```python
from build123d import *

# Parameters (mm, degrees)
F1_DEPTH = 9.525
F2_R     = 5.08
F3_R     = 5.08
F4_R     = 5.08
F5_R     = 7.06815
F6_DEPTH = 75.62089


with BuildPart() as f1:
    # F0 (on Top) → F1 (new body)
    with BuildSketch(Plane.XY):
        Polygon((36.595166, -42.144418), (55.044204, -31.628042), (-28.496206, 58.19229), (-68.840876, 46.343863), (-45.743927, 16.047873), align=None)
    extrude(amount=F1_DEPTH)

    # F2
    f2_edges = [f1.edges().sort_by_distance(p)[0] for p in [
        (-68.840876, 46.343863, 4.7625),
    ]]
    fillet(f2_edges, radius=F2_R)

    # F3
    f3_edges = [f1.edges().sort_by_distance(p)[0] for p in [
        (36.595166, -42.144418, 4.7625),
    ]]
    fillet(f3_edges, radius=F3_R)

    # F4
    f4_edges = [f1.edges().sort_by_distance(p)[0] for p in [
        (55.044204, -31.628042, 4.7625),
    ]]
    fillet(f4_edges, radius=F4_R)

    # F5 (on face) → F6 (cut)
    with BuildSketch(Plane(origin=(0, 0, 0), x_dir=(1, 0, 0), z_dir=(0, 0, -1))):
        with Locations((36.157202, 27.517132)):
            Circle(F5_R)
    extrude(amount=-F6_DEPTH, mode=Mode.SUBTRACT)


solid = f1.part
```
Verification items for the finished model (mm, model axes). Round coordinates to 2 decimals unless told otherwise and drop trailing zeros. Order: outer loops, then holes, each group sorted by start corner. A loop starts at its lowest first (then second) coordinate and runs counter-clockwise, first axis right, second up. Notation, with made-up numbers: (73.5, 35.5) - (98.5, 35.5) arc R19 ccw to (98.5, 66.5) - close; hole circle Ø10 at (-4, -19). An arc over 180 degrees is marked (long way). Use CSV: the item, a comma, the result in double quotes. Start each with the question number.
1) Go/stop test with flat-tipped pins: P1, Ø5, axis at x = 3, z = 1, coming from the -Y side; P2, Ø5, axis at y = 46, z = 6.5, coming from the +X side; P3, Ø22.5, axis at x = 36.16, y = -27.52, coming from the -Z side. Record where each tip stops, or that it passes through.
2) Section check B-B, the plane y = 28.5. Record the cut outline in (x, z) (3 decimals), plus the area to 3 significant figures.
3) Section check C-C, the plane x = -10. Record the cut outline in (y, z) (3 decimals), plus the area to 3 significant figures.
4) Thickness scan on L1, parallel to Y at x = 41, z = 2.75; L2, parallel to Y at x = 36, z = 5.25; L3, parallel to X at y = -30, z = 4.5. Record the ranges inside material, lowest first.
5) Section check A-A, the plane z = 2. Record the cut outline in (x, y).
6) Mould release check, pull along X, two halves, no side actions. Record for faces 1 (the flat face through (44.367, -37.714, 4.696)), 2 (the cylindrical face through (36.681, -41.206, 4.829)), 3 (the cylindrical face through (30.548, -23.216, 4.696)): +X half, -X half, draft (parallel to the pull), parting line (faces both ways), or undercut.
Answers:
1,P1,"stops at y = -20.17"
1,P2,"stops at x = -14.83"
1,P3,"stops at z = 0"
2,outline,"(-55.237, 0) - (-0.88, 0) - (-0.88, 9.525) - (-55.237, 9.525) - close"
2,area,"518 mm²"
3,outline,"(-9.214, 0) - (38.306, 0) - (38.306, 9.525) - (-9.214, 9.525) - close"
3,area,"453 mm²"
4,L1,"y = -39.63 to -32.67, -22.37 to -16.53"
4,L2,"y = -41.13 to -34.58, -20.45 to -11.15"
4,L3,"x = 19.41 to 29.54, 42.77 to 52.02"
5,outline,"(-64.36, 40.47) - (-45.74, 16.05) - (33.96, -40.28) arc R5.08 ccw to (39.4, -40.54) - (49.47, -34.8) arc R5.08 ccw to (50.68, -26.93) - (-28.5, 58.19) - (-61.75, 48.42) arc R5.08 ccw to start; hole circle Ø14.14 at (36.16, -27.52)"
6,face 1,"+X half"
6,face 2,"parting line"
6,face 3,"undercut"
